Verification items for the finished model (mm, model axes). A direction names the side the tool comes from. Coordinates: 2 decimals unless noted, no trailing zeros. Order: outer loops, then holes, each group sorted by start corner. A loop starts at its lowest first (then second) coordinate and runs counter-clockwise, first axis right, second up. Notation, with made-up numbers: M 26,42 L 52,42 A16 ccw 52,49 Z; hole C 3.25,47 d11. An arc over 180 degrees is marked long. Return JSON: item names as keys, results as strings. Group by question number.
Q1. Section check D-D, the plane x = 27.88. Enter the section's corners in (y, z) (3 decimals), then the cut area to 3 significant figures.
Q2. Access from +Z, -Z, +X, -X, +Y, -Y to the whole of each face (thin tool, end or side, straight path). Record for faces 4 (the face through (0, 2, -3.175)), 5 (the face through (-7.5, 0, -2)), 6 (the face through (22, 0, -50)).
Q3. Go/stop test with flat-tipped pins: pin 1 Ø4 at (y, z) = (-1.5, -19.5) entering from +X (3 decimals); pin 2 Ø3.5 at (x, y) = (-3, 1) entering from -Z (3 decimals). Record where each tip stops, or that it passes through.
Q4. Section check B-B, the plane y = 0. Enter the section's corners in (x, z) (3 decimals).
Q5. Section check A-A, the plane x = -2.42. Enter the section's corners in (y, z) (3 decimals).
Q6. Thickness scan on probe 1 along Y at (x, z) = (-2.42, -0.8); probe 2 along Y at (x, z) = (27.88, -51.05); probe 3 along Z at (x, y) = (4, -3) (3 decimals). Record the ranges inside material, lowest first.
Q7. Mould release check, pull along Y, two halves, no side actions. Record for faces 1 (the face through (11.577, -0.105, -49.145)), 2 (the face through (32.725, 1.526, -51.565)), 3 (the face through (-6.6, 6.64, -1.61)): pulls with the +Y half, pulls with the -Y half, needs draft (parallel to the pull), parting line crosses it, or undercut.
Q8. Section check C-C, the plane z = -8. Enter the section's corners in (x, y) (3 decimals), then the cut area to 3 significant figures.
from build123d import *

# Parameters (mm, degrees)
SKETCH1_W                    = 15
SKETCH1_H                    = 15
BASE_FLANGE2_DEPTH           = 3.175
EDGE_FLANGE1_STRIP_W         = 18.7
EDGE_FLANGE1_STRIP_H         = 3.175
EDGE_FLANGE1_STRIP_CUT_DEPTH = 15
EDGE_FLANGE1_DEPTH           = 15
EDGE_FLANGE2_STRIP_W         = 18.7
EDGE_FLANGE2_STRIP_H         = 3.175
EDGE_FLANGE2_STRIP_CUT_DEPTH = 15
EDGE_FLANGE2_DEPTH           = 15
SKETCH18_R                   = 2.54
CUT_EXTRUDE1_DEPTH           = 65.374533979
SKETCH19_R                   = 5.08
CUT_EXTRUDE2_DEPTH           = 62.777827738
FILLET1_R                    = 3


# Sheet-metal steps are written as plain solids
with BuildPart() as part:
    # Sketch1 → Base-Flange2 (new body)
    with BuildSketch(Plane.XY):
        Rectangle(SKETCH1_W, SKETCH1_H)
    extrude(amount=-BASE_FLANGE2_DEPTH)

    # Edge-Flange1 strip (across the edge) → Edge-Flange1 strip cut (cut)
    with BuildSketch(Plane(origin=(7.5, 7.5, -3.175), x_dir=(-1, 0, 0), z_dir=(0, -1, 0))):
        with Locations((-6.35, -1.5875)):
            Rectangle(EDGE_FLANGE1_STRIP_W, EDGE_FLANGE1_STRIP_H)
    extrude(amount=EDGE_FLANGE1_STRIP_CUT_DEPTH, mode=Mode.SUBTRACT)

    # Edge-Flange1 section (across the edge) → Edge-Flange1 (add)
    with BuildSketch(Plane(origin=(7.5, 7.5, -3.175), x_dir=(-1, 0, 0), z_dir=(0, -1, 0))):
        with BuildLine():
            Line((-3.175, 3), (-3.175, 46.825))
            Line((-3.175, 46.825), (0, 46.825))
            Line((0, 46.825), (0, 3))
            ThreePointArc((0, 3), (0.878679656, 0.878679656), (3, 0))
            Line((3, 0), (3, -3.175))
            ThreePointArc((3, -3.175), (-1.366384374, -1.366384374), (-3.175, 3))
        make_face()
    extrude(amount=EDGE_FLANGE1_DEPTH)

    # Edge-Flange2 strip (across the edge) → Edge-Flange2 strip cut (cut)
    with BuildSketch(Plane(origin=(10.675, -7.5, -50), x_dir=(0, 0, 1), z_dir=(0, 1, 0))):
        with Locations((-6.35, -1.5875)):
            Rectangle(EDGE_FLANGE2_STRIP_W, EDGE_FLANGE2_STRIP_H)
    extrude(amount=EDGE_FLANGE2_STRIP_CUT_DEPTH, mode=Mode.SUBTRACT)

    # Edge-Flange2 section (across the edge) → Edge-Flange2 (add)
    with BuildSketch(Plane(origin=(10.675, -7.5, -50), x_dir=(0, 0, 1), z_dir=(0, 1, 0))):
        with BuildLine():
            Line((-3.175, 3), (-3.175, 24.825))
            Line((-3.175, 24.825), (0, 24.825))
            Line((0, 24.825), (0, 3))
            ThreePointArc((0, 3), (0.878679656, 0.878679656), (3, 0))
            Line((3, 0), (3, -3.175))
            ThreePointArc((3, -3.175), (-1.366384374, -1.366384374), (-3.175, 3))
        make_face()
    extrude(amount=EDGE_FLANGE2_DEPTH)

    # Sketch18 → Cut-Extrude1 (cut, through all)
    with BuildSketch(Plane.XY):
        with Locations((-2.42, 0)):
            Circle(SKETCH18_R)
    extrude(amount=-CUT_EXTRUDE1_DEPTH, mode=Mode.SUBTRACT)

    # Sketch19 → Cut-Extrude2 (cut, through all)
    with BuildSketch(Plane.XY.offset(-50)):
        with Locations((27.88, 0)):
            Circle(SKETCH19_R)
    extrude(amount=-CUT_EXTRUDE2_DEPTH, mode=Mode.SUBTRACT)

    # Fillet1
    fillet1_edges = [part.edges().sort_by_distance(p)[0] for p in [
        (35.5, -7.5, -51.5875),
        (35.5, 7.5, -51.5875),
        (-7.5, -7.5, -1.5875),
        (-7.5, 7.5, -1.5875),
    ]]
    fillet(fillet1_edges, radius=FILLET1_R)


solid = part.part
Numbers:
{
 "1": {"outline": "M -7.5,-53.175 L -5.08,-53.175 L -5.08,-50 L -7.5,-50 Z; M 5.08,-53.175 L 7.5,-53.175 L 7.5,-50 L 5.08,-50 Z", "area": "15.4 mm2"},
 "2": {"face 4": "-Z, -X, +Y, -Y", "face 5": "+Z, -Z, -X, +Y, -Y", "face 6": "+Z, +X, +Y, -Y"},
 "3": {"pin 1": "stops at x = 10.675", "pin 2": "stops at z = -3.175"},
 "4": {"outline": "M -7.5,-3.175 L -4.96,-3.175 L -4.96,0 L -7.5,0 Z; M 0.12,-3.175 L 4.5,-3.175 A3 cw 7.5,-6.175 L 7.5,-47 A6.175 ccw 13.675,-53.175 L 22.8,-53.175 L 22.8,-50 L 13.675,-50 A3 cw 10.675,-47 L 10.675,-6.175 A6.175 ccw 4.5,0 L 0.12,0 Z; M 32.96,-53.175 L 35.5,-53.175 L 35.5,-50 L 32.96,-50 Z"},
 "5": {"outline": "M -7.5,-3.175 L -2.54,-3.175 L -2.54,0 L -7.5,0 Z; M 2.54,-3.175 L 7.5,-3.175 L 7.5,0 L 2.54,0 Z"},
 "6": {"probe 1": "y = -7.5 to -2.54, 2.54 to 7.5", "probe 2": "y = -7.5 to -5.08, 5.08 to 7.5", "probe 3": "z = -3.175 to 0"},
 "7": {"face 1": "needs draft", "face 2": "undercut", "face 3": "pulls with the +Y half"},
 "8": {"outline": "M 7.5,-7.5 L 10.675,-7.5 L 10.675,7.5 L 7.5,7.5 Z", "area": "47.6 mm2"}
}
